from build123d import *

# Parameters (mm, degrees)
CUT_EXTRUDE6_DEPTH  = 75
CUT_EXTRUDE7_DEPTH  = 48
SKETCH11_W          = 39
SKETCH11_H          = 22
CUT_EXTRUDE8_DEPTH  = 56
SKETCH14_W          = 50.821005264
SKETCH14_H          = 8.659157084
SKETCH14_W_2        = 55.150583806
SKETCH14_H_2        = 9.071497897
CUT_EXTRUDE11_DEPTH = 90
SKETCH15_W          = 52.591955303
SKETCH15_H          = 17.949813053
CUT_EXTRUDE12_DEPTH = 100


with BuildPart() as part:
    # Sketch1 → Revolve1 (revolve)
    with BuildSketch(Plane(origin=(0, 0, 0), x_dir=(1, 0, 0), z_dir=(0, 1, 0))):
        Polygon((-14.084428196, 16.517586435), (-1.084428196, 16.517586435), (-1.084428196, -3.482413565), (17.915571804, -24.482413565), (17.915571804, -73.482413565), (-14.084428196, -73.482413565), align=None)
    revolve(axis=Axis((-14.084428196, 0, 73.482413565), (0, 0, -1)))

    # Sketch7 → Cut-Extrude6 (cut)
    with BuildSketch(Plane.XY.offset(73.482413565)):
        with BuildLine():
            ThreePointArc((8.542988801, 22.627416998), (-1.838558361, 29.56414504), (-14.084428196, 32))
            Line((-14.084428196, 32), (-14.084428196, 22.627416998))
            Line((-14.084428196, 22.627416998), (8.542988801, 22.627416998))
        make_face()
        with BuildLine():
            Line((-14.084428196, 22.627416998), (-14.084428196, 32))
            ThreePointArc((-14.084428196, 32), (-26.330298032, 29.56414504), (-36.711845194, 22.627416998))
            Line((-36.711845194, 22.627416998), (-14.084428196, 22.627416998))
        make_face()
        with BuildLine():
            Line((-36.747904754, 0), (-36.747904754, 22.591299881))
            ThreePointArc((-36.747904754, 22.591299881), (-43.658329274, 12.222290091), (-46.084428196, 0))
            Line((-46.084428196, 0), (-36.747904754, 0))
        make_face()
        with BuildLine():
            Line((-36.747904754, -22.591299881), (-36.747904754, 0))
            Line((-36.747904754, 0), (-46.084428196, 0))
            ThreePointArc((-46.084428196, 0), (-43.658329274, -12.222290091), (-36.747904754, -22.591299881))
        make_face()
        with BuildLine():
            Line((-14.084428196, -32), (-14.084428196, -22.591299881))
            Line((-14.084428196, -22.591299881), (-36.747904754, -22.591299881))
            ThreePointArc((-36.747904754, -22.591299881), (-26.353869989, -29.554370203), (-14.084428196, -32))
        make_face()
        with BuildLine():
            ThreePointArc((17.915571804, 0), (15.479716844, 12.245869836), (8.542988801, 22.627416998))
            Line((8.542988801, 22.627416998), (8.542988801, 0))
            Line((8.542988801, 0), (17.915571804, 0))
        make_face()
        with BuildLine():
            Line((17.915571804, 0), (8.542988801, 0))
            Line((8.542988801, 0), (8.542988801, -22.591299881))
            Line((8.542988801, -22.591299881), (-14.084428196, -22.591299881))
            Line((-14.084428196, -22.591299881), (-14.084428196, -32))
            ThreePointArc((-14.084428196, -32), (8.542988801, -22.627416998), (17.915571804, 0))
        make_face()
    extrude(amount=-CUT_EXTRUDE6_DEPTH, mode=Mode.SUBTRACT)

    # Sketch10 → Cut-Extrude7 (cut)
    with BuildSketch(Plane(origin=(0, 0, -16.517586435), x_dir=(-1, 0, 0), z_dir=(0, 0, -1))):
        with BuildLine():
            ThreePointArc((24.584428196, 0), (21.509049399, 7.424621202), (14.084428196, 10.5))
            Line((14.084428196, 10.5), (14.084428196, 0))
            Line((14.084428196, 0), (24.584428196, 0))
        make_face()
        with BuildLine():
            Line((14.084428196, 0), (14.084428196, 10.5))
            ThreePointArc((14.084428196, 10.5), (6.659806994, 7.424621202), (3.584428196, 0))
            Line((3.584428196, 0), (14.084428196, 0))
        make_face()
        with BuildLine():
            Line((24.584428196, 0), (14.084428196, 0))
            Line((14.084428196, 0), (14.084428196, -10.5))
            ThreePointArc((14.084428196, -10.5), (21.509049399, -7.424621202), (24.584428196, 0))
        make_face()
        with BuildLine():
            Line((14.084428196, -10.5), (14.084428196, 0))
            Line((14.084428196, 0), (3.584428196, 0))
            ThreePointArc((3.584428196, 0), (6.659806994, -7.424621202), (14.084428196, -10.5))
        make_face()
    extrude(amount=-CUT_EXTRUDE7_DEPTH, mode=Mode.SUBTRACT)

    # Sketch11 → Cut-Extrude8 (cut)
    with BuildSketch(Plane.XY.offset(73.482413565)):
        with Locations((-14.247904754, 0.565694089)):
            Rectangle(SKETCH11_W, SKETCH11_H)
    extrude(amount=-CUT_EXTRUDE8_DEPTH, mode=Mode.SUBTRACT)

    # Sketch14 → Cut-Extrude11 (cut)
    with BuildSketch(Plane.XY.offset(73.482413565)):
        with Locations((-14.154000578, 19.895272631)):
            Rectangle(SKETCH14_W, SKETCH14_H)
        with Locations((-15.391023019, -18.97005486)):
            Rectangle(SKETCH14_W_2, SKETCH14_H_2)
    extrude(amount=-CUT_EXTRUDE11_DEPTH, mode=Mode.SUBTRACT)

    # Sketch15 → Cut-Extrude12 (cut)
    with BuildSketch(Plane(origin=(0, 0, -16.517586435), x_dir=(-1, 0, 0), z_dir=(0, 0, -1))):
        with Locations((12.823626237, 8.974906526)):
            Rectangle(SKETCH15_W, SKETCH15_H)
    extrude(amount=-CUT_EXTRUDE12_DEPTH, mode=Mode.SUBTRACT)


solid = part.part
Input: part model. Units: mm. Frame: model coordinates. A direction names the side the tool comes from. Give positions to 0.01 mm unless a question says otherwise; leave off trailing zeros. Order: outer loops, then holes, each group sorted by start corner. A loop starts at its lowest first (then second) coordinate and runs counter-clockwise, first axis right, second up.
Q1. Contact query for flat-ended pins moving along their axis: pin 1 Ø5 at (x, y) = (-1, -4.5) entering from +Z; pin 2 Ø4 at (x, z) = (-7.5, 24.5) entering from +Y; pin 3 Ø1 at (x, z) = (-17.5, 7.5) entering from +Y. Output: stop coordinate, or through.
Checked values:
pin 1: stops at z = 17.48
pin 2: stops at y = -10.43
pin 3: stops at y = -9.74
Q2. Set-up query: faces 1 (the flat face through (6, 0, 25)), 2 (the flat face through (-15, -10.434, 46)), 3 (the cylindrical face through (-14, -13, -6)). Return all of +Z, -Z, +X, -X, +Y, -Y with unobstructed straight access to the full face (end or side cutting, diameter ignored); none if empty.
Checked values:
face 1: +Z, -Z, +X, -X, +Y
face 2: +Z, +Y
face 3: -Z, -Y
Q3. Section A-A on z = 22. Output: boundary loops of the cut face in (x, y).
Checked values:
outline: (-36.75, -14.43) - (8.54, -14.43) - (8.54, 0) - (5.25, 0) - (5.25, -10.43) - (-12.91, -10.43) arc R10.5 cw to (-15.26, -10.43) - (-33.75, -10.43) - (-33.75, 0) - (-36.75, 0) - close
Q4. Section C-C on z = 10.5. Output: boundary loops of the cut face in (x, y), and give its area (3 significant figures).
Checked values:
outline: (-33.43, 0) arc R19.35 ccw to (-26.97, -14.43) - (-1.2, -14.43) arc R19.35 ccw to (5.26, 0) - (-3.58, 0) arc R10.5 cw to (-24.58, 0) - close
area: 328 mm2
Q5. Ray query, probe 1 along X at (y, z) = (-10, 24); probe 2 along Y at (x, z) = (-23, 54.5); probe 3 along X at (y, z) = (-9.25, 15.5). Return the intervals inside material, ascending.
Checked values:
probe 1: x = -36.75 to -33.75, 5.25 to 8.54
probe 2: y = -14.43 to -10.43
probe 3: x = -36.09 to -19.05, -9.12 to 7.92
Q6. Section B-B on z = 32.5. Output: boundary loops of the cut face in (x, y), and give its area (3 significant figures).
Checked values:
outline: (-36.75, -14.43) - (8.54, -14.43) - (8.54, 0) - (5.25, 0) - (5.25, -10.43) - (-33.75, -10.43) - (-33.75, 0) - (-36.75, 0) - close
area: 247 mm2
